Design review of the part shown in the three views and the two pictorial views. Dimensions are in mm from the part's minimum x, y and z. Give positions to 0.01 mm unless a question says otherwise; leave off trailing zeros. Loops run counter-clockwise (first coordinate to the right, second up) from the corner with the lowest first, then second, coordinate; pieces in that order, holes last.
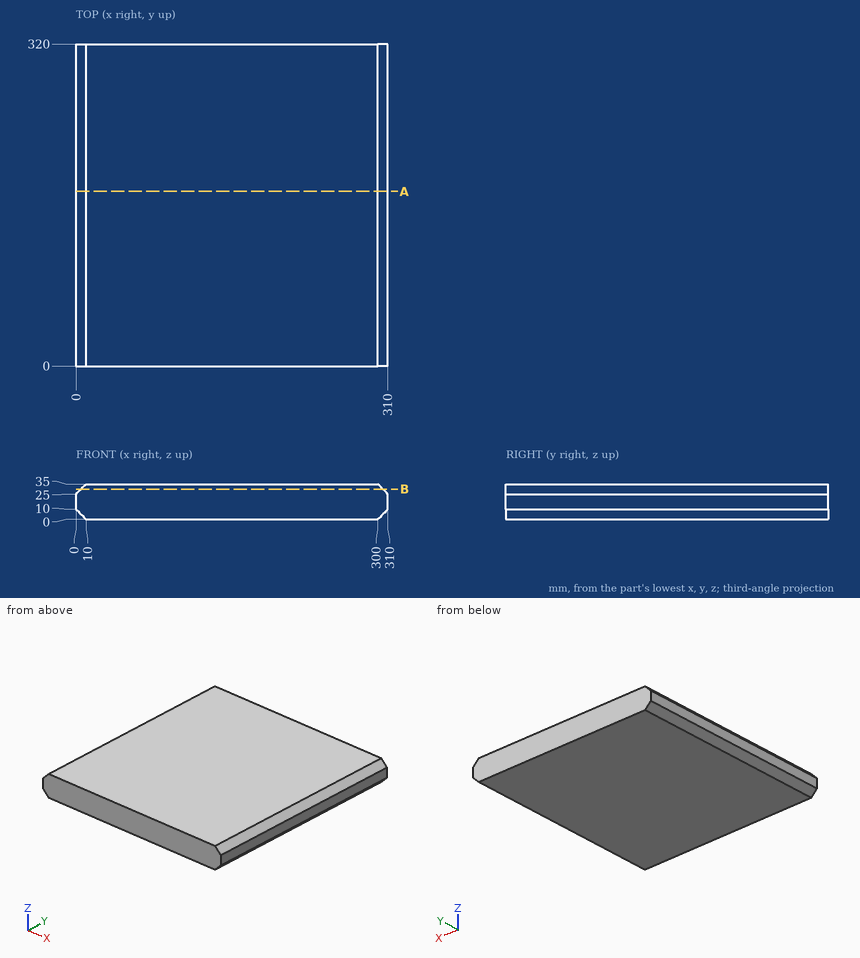
Q1. Consider section A-A on y = 173.5. Give the boundary of the cut face in (x, z).
Answers:
outline: (0, 10) - (10, 0) - (300, 0) - (310, 10) - (310, 25) - (300, 35) - (10, 35) - (0, 25) - close
Q2. For pin 1 Ø4 at (y, z) = (259, 26) entering from +X, flat-tipped, find the tip position at first contact; note if it passes through.
Answers:
pin 1: stops at x = 310
Q3. Consider section B-B on z = 30. Give the boundary of the cut face in (x, y), plus the area to 3 significant figures.
Answers:
outline: (5, 0) - (305, 0) - (305, 320) - (5, 320) - close
area: 96,000 mm2
Q4. For probe 1 along X at (y, z) = (301.5, 7); probe 2 along X at (y, z) = (245, 32.5), list the stretches that pass through material, from the lowest coordinate up.
Answers:
probe 1: x = 3 to 307
probe 2: x = 7.5 to 302.5
